Verification items for the finished model (mm, model axes). A direction names the side the tool comes from. Round coordinates to 2 decimals unless told otherwise and drop trailing zeros. Order: outer loops, then holes, each group sorted by start corner. A loop starts at its lowest first (then second) coordinate and runs counter-clockwise, first axis right, second up. Notation, with made-up numbers: (5.25, -13) -> (58.25, -13) arc R18 ccw to (58.25, -9) -> close; hole circle Ø6 at (4.5, 64). An arc over 180 degrees is marked (long way). Return JSON: item names as keys, results as strings. Group by question number.
Item 1: Access from +Z, -Z, +X, -X, +Y, -Y to the whole of each face (thin tool, end or side, straight path). Record for faces 1 (the flat face through (0, -11, 19.05)), 2 (the flat face through (0, 7.368, 66)), 3 (the cylindrical face through (-10.413, 0.115, 66.008)), 4 (the flat face through (0, -7.368, 66)).
Item 2: Sectioned sample at C-C on z = 84. Record the cut outline in (x, y).
Item 3: Scan lines: probe 1 along Z at (x, y) = (-23, 2.5); probe 2 along Y at (x, z) = (3, 81.5); probe 3 along X at (y, z) = (23, 8.5). Record each from-to range of solid material in increasing order. Write a range as from..to.
Item 4: Sectioned sample at D-D on y = -12. Record the cut outline in (x, z), plus the area to 3 significant figures.
Item 5: Sectioned sample at A-A on y = 0. Record the cut outline in (x, z).
Item 6: Depth check by flat-ended pin: pin 1 Ø6 at (x, z) = (7, 45) entering from -Y; pin 2 Ø12 at (x, z) = (19, 88) entering from +Y; pin 3 Ø3 at (y, z) = (1, 101) entering from +X; pin 4 Ø1 at (x, y) = (3.5, 19) entering from +Z. Enter the tip coordinate at first touch or a pass-through.
Item 7: Sectioned sample at B-B on x = 0. Record the cut outline in (y, z).
```python
from build123d import *

# Parameters (mm, degrees)
BOSS_EXTRUDE1_DEPTH = 114.3
SKETCH3_R           = 25.401969389
BOSS_EXTRUDE2_DEPTH = 19.05


with BuildPart() as part:
    # Sketch1 → Boss-Extrude1 (new body)
    with BuildSketch(Plane.XY):
        with BuildLine():
            Line((-7.359452383, -7.368165079), (7.359452383, -7.368165079))
            ThreePointArc((7.359452383, -7.368165079), (10.414, 0), (7.359452383, 7.368165079))
            Line((7.359452383, 7.368165079), (-7.359452383, 7.368165079))
            ThreePointArc((-7.359452383, 7.368165079), (-10.414, 0), (-7.359452383, -7.368165079))
        make_face()
    extrude(amount=BOSS_EXTRUDE1_DEPTH)

    # Sketch3 → Boss-Extrude2 (add)
    with BuildSketch(Plane(origin=(0, 0, 0), x_dir=(-1, 0, 0), z_dir=(0, 0, -1))):
        Circle(SKETCH3_R)
    extrude(amount=-BOSS_EXTRUDE2_DEPTH)


solid = part.part
```
Recorded:
{
 "1": {"face 1": "+Z", "face 2": "+Z, +X, -X, +Y", "face 3": "+Z, -X", "face 4": "+Z, +X, -X, -Y"},
 "2": {"outline": "(-7.36, -7.37) -> (7.36, -7.37) arc R10.41 ccw to (7.36, 7.37) -> (-7.36, 7.37) arc R10.41 ccw to start"},
 "3": {"probe 1": "0..19.05", "probe 2": "-7.37..7.37", "probe 3": "-10.78..10.78"},
 "4": {"outline": "(-22.39, 0) -> (22.39, 0) -> (22.39, 19.05) -> (-22.39, 19.05) -> close", "area": "853 mm²"},
 "5": {"outline": "(-25.4, 0) -> (25.4, 0) -> (25.4, 19.05) -> (10.41, 19.05) -> (10.41, 114.3) -> (-10.41, 114.3) -> (-10.41, 19.05) -> (-25.4, 19.05) -> close"},
 "6": {"pin 1": "y = -7.37", "pin 2": "through", "pin 3": "x = 10.41", "pin 4": "z = 19.05"},
 "7": {"outline": "(-25.4, 0) -> (25.4, 0) -> (25.4, 19.05) -> (7.37, 19.05) -> (7.37, 114.3) -> (-7.37, 114.3) -> (-7.37, 19.05) -> (-25.4, 19.05) -> close"}
}
